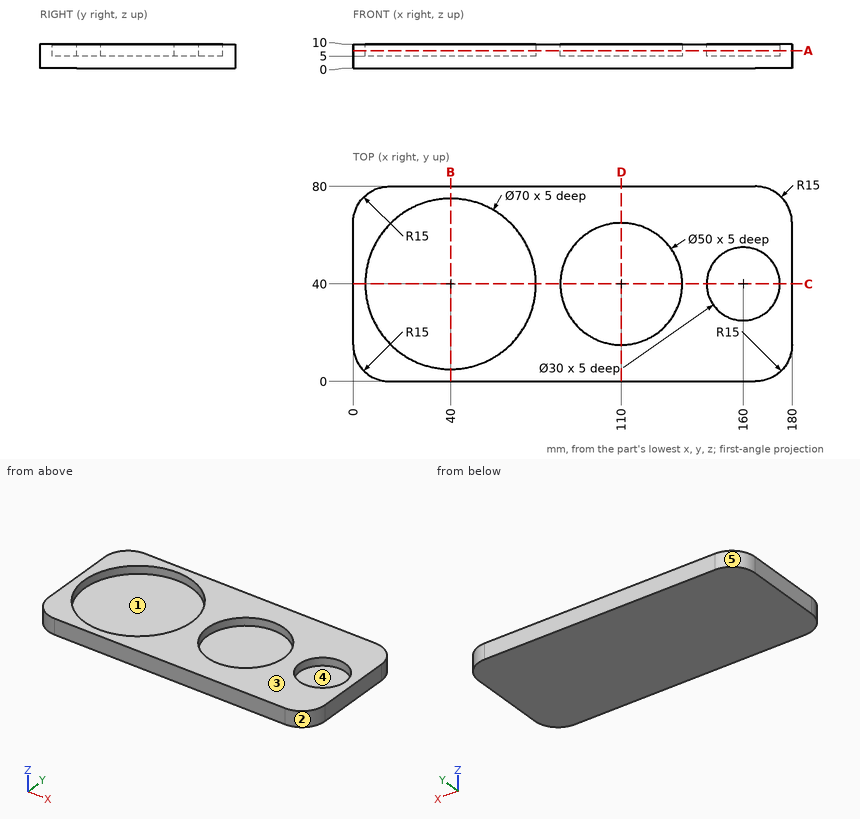
Can you work these out from the drawing? Everything is in mm from the part's minimum corner. A direction names the side the tool comes from. Round coordinates to 2 decimals unless told otherwise and drop trailing zeros. Order: outer loops, then holes, each group sorted by start corner. A loop starts at its lowest first (then second) coordinate and runs counter-clockwise, first axis right, second up. Notation, with made-up numbers: (-36.75, 65.25) -> (-27.75, 65.25) arc R9 ccw to (-27.75, 80.25) -> close; hole circle Ø9 at (86, -26.5). An arc over 180 degrees is marked (long way). Return JSON: item names as keys, results as strings. Group by question number.
1. If we section it at D-D, the plane x = 110: Write out the boundary of the cut face in (y, z).
2. Which directions (+Z, -Z, +X, -X, +Y, -Y) give clear straight access to the entire face, cutting with the end or side of a thin tool? Please do the marked faces 1 and 2.
3. If we section it at C-C, the plane y = 40: Write out the boundary of the cut face in (x, z).
4. I need wall thicknesses on line 1 (Y direction, x = 160, z = 7.95); line 2 (X direction, y = 39, z = 5.25); line 3 (X direction, y = 38, z = 8.5). Which ranges of each line are inside material? Lowest first, please. Write a range as [from, to].
5. We'd pull the mould along Y, two halves only. Please class the marked faces 3, 4 and 5: released by +Y, released by -Y, zero draft, split by the parting line, or undercut.
6. If we section it at A-A, the plane z = 7.25: Write out the boundary of the cut face in (x, y).
7. If we section it at B-B, the plane x = 40: Write out the boundary of the cut face in (y, z).
8. Will this pin go through, and if not, where does the flat tip stop? pin 1 (15 mm diameter, centred on x = 104.5, y = 28.5, fed in from +Z).
Output values:
{
 "1": {"outline": "(0, 0) -> (80, 0) -> (80, 10) -> (65, 10) -> (65, 5) -> (15, 5) -> (15, 10) -> (0, 10) -> close"},
 "2": {"face 1": "+Z", "face 2": "+Z, -Z, +X, -Y"},
 "3": {"outline": "(0, 0) -> (180, 0) -> (180, 10) -> (175, 10) -> (175, 5) -> (145, 5) -> (145, 10) -> (135, 10) -> (135, 5) -> (85, 5) -> (85, 10) -> (75, 10) -> (75, 5) -> (5, 5) -> (5, 10) -> (0, 10) -> close"},
 "4": {"line 1": "[0, 25], [55, 80]", "line 2": "[0, 5.01], [74.99, 85.02], [134.98, 145.03], [174.97, 180]", "line 3": "[0, 5.06], [74.94, 85.08], [134.92, 145.13], [174.87, 180]"},
 "5": {"face 3": "zero draft", "face 4": "undercut", "face 5": "released by +Y"},
 "6": {"outline": "(0, 15) arc R15 ccw to (15, 0) -> (165, 0) arc R15 ccw to (180, 15) -> (180, 65) arc R15 ccw to (165, 80) -> (15, 80) arc R15 ccw to (0, 65) -> close; hole circle Ø70 at (40, 40); hole circle Ø50 at (110, 40); hole circle Ø30 at (160, 40)"},
 "7": {"outline": "(0, 0) -> (80, 0) -> (80, 10) -> (75, 10) -> (75, 5) -> (5, 5) -> (5, 10) -> (0, 10) -> close"},
 "8": {"pin 1": "z = 5"}
}
